from build123d import *

# Parameters (mm, degrees)
BOSS_EXTRUDE1_DEPTH = 190.5
SKETCH2_W           = 25.4
SKETCH2_H           = 6.35
BOSS_EXTRUDE2_DEPTH = 6.35
LPATTERN1_COUNT     = 3
LPATTERN1_PITCH     = 50.8
BOSS_EXTRUDE3_DEPTH = 6.35
LPATTERN2_COUNT     = 2
LPATTERN2_PITCH     = 31.75
SKETCH4_R           = 2.7305
CUT_EXTRUDE1_DEPTH  = 212.762427449
CUT_EXTRUDE2_DEPTH  = 212.762427449
SKETCH6_R           = 2.0955
CUT_EXTRUDE3_DEPTH  = 212.762427449


with BuildPart() as part:
    # Sketch1 → Boss-Extrude1 (new body)
    with BuildSketch(Plane.XY):
        Polygon((-73.638100193, 43.604904797), (-37.717075708, 7.683880312), (-33.226947648, 12.174008373), (-69.147972132, 48.095032857), align=None)
    extrude(amount=BOSS_EXTRUDE1_DEPTH)

    # Sketch2 → Boss-Extrude2 (add)
    with BuildSketch(Plane(origin=(-58.621502495, 58.621502495, 0), x_dir=(0, 0, 1), z_dir=(-0.7071067811865471, 0.7071067811865479, 0))):
        with Locations((152.4, -18.061676125)):
            Rectangle(SKETCH2_W, SKETCH2_H)
    boss_extrude2 = extrude(amount=BOSS_EXTRUDE2_DEPTH)

    # LPattern1: Boss-Extrude2 ×3
    with Locations(*[(0, 0, -i * LPATTERN1_PITCH) for i in range(1, LPATTERN1_COUNT)]):
        add(boss_extrude2)

    # Sketch3 → Boss-Extrude3 (add)
    with BuildSketch(Plane(origin=(0, 0, 0), x_dir=(-1, 0, 0), z_dir=(0, 0, -1))):
        Polygon((73.638100193, 43.604904797), (64.657844072, 34.624648676), (60.167716011, 39.114776736), (69.147972132, 48.095032857), align=None)
    boss_extrude3 = extrude(amount=BOSS_EXTRUDE3_DEPTH)

    # LPattern2: Boss-Extrude3 ×2
    with Locations(*[Vector(0.7071067811865476, -0.7071067811865476, 0) * (i * LPATTERN2_PITCH) for i in range(1, LPATTERN2_COUNT)]):
        add(boss_extrude3)

    # Sketch4 → Cut-Extrude1 (cut, through all)
    with BuildSketch(Plane(origin=(-10.526469638, -10.526469638, 0), x_dir=(0, 0, -1), z_dir=(0.7071067811865482, 0.7071067811865468, 0))):
        with Locations(Location((-159.0375, 57.503323875, 0), (0, 0, 90))):
            Circle(SKETCH4_R)
    extrude(amount=-CUT_EXTRUDE1_DEPTH, mode=Mode.SUBTRACT)

    # Sketch5 → Cut-Extrude2 (cut, through all)
    with BuildSketch(Plane(origin=(-10.526469638, -10.526469638, 0), x_dir=(0, 0, -1), z_dir=(0.7071067811865487, 0.7071067811865465, 0))):
        Polygon((-175.6664, 82.903323875), (-179.9336, 82.903323875), (-179.9336, 74.140323875), (-182.245, 74.140323875), (-182.245, 70.965323875), (-179.9336, 70.965323875), (-179.9336, 67.663323875), (-175.6664, 67.663323875), (-175.6664, 70.965323875), (-173.355, 70.965323875), (-173.355, 74.140323875), (-175.6664, 74.140323875), align=None)
        Polygon((-74.0664, 82.903323875), (-78.3336, 82.903323875), (-78.3336, 74.140323875), (-80.645, 74.140323875), (-80.645, 70.965323875), (-78.3336, 70.965323875), (-78.3336, 67.663323875), (-74.0664, 67.663323875), (-74.0664, 70.965323875), (-71.755, 70.965323875), (-71.755, 74.140323875), (-74.0664, 74.140323875), align=None)
        Polygon((-13.7414, 82.903323875), (-18.0086, 82.903323875), (-18.0086, 74.140323875), (-20.32, 74.140323875), (-20.32, 70.965323875), (-18.0086, 70.965323875), (-18.0086, 67.663323875), (-13.7414, 67.663323875), (-13.7414, 70.965323875), (-11.43, 70.965323875), (-11.43, 74.140323875), (-13.7414, 74.140323875), align=None)
    extrude(amount=-CUT_EXTRUDE2_DEPTH, mode=Mode.SUBTRACT)

    # Sketch6 → Cut-Extrude3 (cut, through all)
    with BuildSketch(Plane(origin=(-15.016597698, -15.016597698, 0), x_dir=(0, 0, 1), z_dir=(-0.7071067811865486, -0.7071067811865465, 0))):
        with Locations(Location((152.42060291, 86.078323875, 0), (0, 0, 270))):
            Circle(SKETCH6_R)
        with Locations(Location((50.82060291, 86.078323875, 0), (0, 0, 270))):
            Circle(SKETCH6_R)
    extrude(amount=-CUT_EXTRUDE3_DEPTH, mode=Mode.SUBTRACT)


solid = part.part
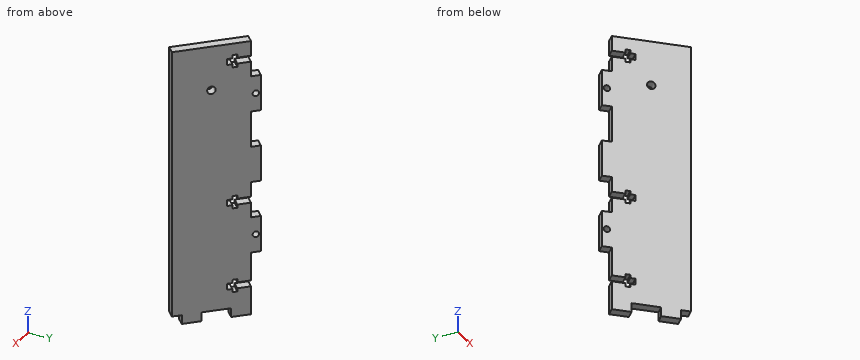
The listing builds one solid part. Answer for the finished solid, in the listing's coordinates (mm). Coordinates: 2 decimals unless noted, no trailing zeros. Order: outer loops, then holes, each group sorted by start corner. A loop starts at its lowest first (then second) coordinate and runs counter-clockwise, first axis right, second up.
Q1. A cutting plane is placed at A-A, the plane z = 127. Write down the section's boundary in (x, y).
Q2. Given P1, Ø8, axis at y = 47.5, z = 68, coming from the +X side; P2, Ø12, axis at x = -53, y = 32.5, coming from the -Z side; P3, Ø10, axis at y = 33, z = 108.5, coming from the +X side, each flat-ended and moving along its own axis, determine where each tip first touches the part or whether it passes through.
Q3. Consider line 1 (Z direction, x = -70, y = 42); line 2 (Z direction, x = -59.5, y = 34); line 3 (X direction, y = 45.5, z = 21). Determine where each line is inside the solid, lowest interval first.
Q4. A cutting plane is placed at B-B, the plane x = -40. Write down the section's boundary in (y, z), and give its area (3 significant figures).
Answers follow:
1. outline: (-73.64, 43.6) - (-37.72, 7.68) - (-33.23, 12.17) - (-69.15, 48.1) - close
2. P1: stops at x = -64.55
2. P2: stops at z = 0
2. P3: stops at x = -49.05
3. line 1: z = -6.35 to 13.74, 18.01 to 74.07, 78.33 to 175.67, 179.93 to 190.5
3. line 2: z = 0 to 190.5
3. line 3: x = -71.74 to -66.55
4. outline: (9.97, 0) - (14.38, 0) - (14.38, -6.35) - (18.95, -6.35) - (18.95, 190.5) - (9.97, 190.5) - close
4. area: 1,740 mm2
